```python
from build123d import *
from build123d import SkipClean  # not in build123d's __all__

# Parameters (mm, degrees)
F0_W     = 48
F0_H     = 30
F0_R     = 1.5
F0_W_2   = 14
F0_H_2   = 5
F0_W_3   = 5
F0_H_3   = 11
F0_R_2   = 3
F0_R_3   = 1.75
F1_DEPTH = 6
F2_DEPTH = 2
F5_DEPTH = 12
F6_DEPTH = 12.001
F7_DEPTH = 30.001


with BuildPart() as f1:
    # F0 (on Front) → F1 (new body)
    with BuildSketch(Plane.XZ):
        Rectangle(F0_W, F0_H)
        with Locations((-15.5, -11)):
            Circle(F0_R, mode=Mode.SUBTRACT)
        with Locations((-6, -5)):
            Rectangle(F0_W_2, F0_H_2, mode=Mode.SUBTRACT)
        with Locations((3.5, -11)):
            Circle(F0_R, mode=Mode.SUBTRACT)
        with Locations((9.5, -5.5)):
            Rectangle(F0_W_3, F0_H_3, mode=Mode.SUBTRACT)
        with Locations((-18, 8)):
            Circle(F0_R_2, mode=Mode.SUBTRACT)
        with Locations((8, 8)):
            Circle(F0_R_2, mode=Mode.SUBTRACT)
        with Locations((-6, -5)):
            Rectangle(F0_W_2, F0_H_2)
        with Locations((9.5, -5.5)):
            Rectangle(F0_W_3, F0_H_3)
        with Locations((8, 8)):
            Circle(F0_R_2)
        with Locations((8, 8)):
            Circle(F0_R_3, mode=Mode.SUBTRACT)
        with Locations((-18, 8)):
            Circle(F0_R_2)
        with Locations((-18, 8)):
            Circle(F0_R_3, mode=Mode.SUBTRACT)
    extrude(amount=-F1_DEPTH)

    # F0 (on Front) → F2 (cut)
    with BuildSketch(Plane.XZ):
        with Locations((9.5, -5.5)):
            Rectangle(F0_W_3, F0_H_3)
        with Locations((-6, -5)):
            Rectangle(F0_W_2, F0_H_2)
        with Locations((-18, 8)):
            Circle(F0_R_2)
        with Locations((-18, 8)):
            Circle(F0_R_3, mode=Mode.SUBTRACT)
        with Locations((8, 8)):
            Circle(F0_R_2)
        with Locations((8, 8)):
            Circle(F0_R_3, mode=Mode.SUBTRACT)
    extrude(amount=-F2_DEPTH, mode=Mode.SUBTRACT)

    # F4 (on face) → F5 (join)
    with BuildSketch(Plane.XY.offset(15)):
        with BuildLine():
            Line((-24, 12), (-24, 6))
            Line((-24, 6), (-11.2915026221, 6))
            ThreePointArc((-11.2915026221, 6), (-13.2915026221, 8.7084973779), (-14, 12))
            Line((-14, 12), (-24, 12))
        make_face()
        with BuildLine():
            ThreePointArc((2, 12), (1.2915026221, 8.7084973779), (-0.7084973779, 6))
            Line((-0.7084973779, 6), (24, 6))
            Line((24, 6), (24, 12))
            Line((24, 12), (2, 12))
        make_face()
    extrude(amount=-F5_DEPTH)

    # F0 (on Front) → F6 (cut, through all)
    with BuildSketch(Plane.XZ):
        with Locations((-18, 8)):
            Circle(F0_R_3)
        with Locations((8, 8)):
            Circle(F0_R_3)
    extrude(amount=-F6_DEPTH, mode=Mode.SUBTRACT)

    # F4 (on face) → F7 (cut, through all)
    with BuildSketch(Plane.XY.offset(15)):
        with BuildLine():
            Line((-0.7084973779, 6), (-11.2915026221, 6))
            ThreePointArc((-11.2915026221, 6), (-6, 4), (-0.7084973779, 6))
        make_face()
    with SkipClean():  # cleaning this boolean's faces spoils the solid; the shape is the same uncleaned
        extrude(amount=-F7_DEPTH, mode=Mode.SUBTRACT)


solid = f1.part
```
Read the model definition and answer for the solid it produces. Units are mm, in the model's axes. A direction names the side the tool comes from. Round coordinates to 2 decimals unless told otherwise and drop trailing zeros. Write each loop counter-clockwise with the first axis right and the second up, starting at its lowest first coordinate (ties: lowest second). Pieces come first, ordered by that corner, then holes. Notation, with made-up numbers: (2.5, 8.5) -> (10.5, 8.5) arc R30 cw to (10.5, 33.5) -> close; hole circle Ø10 at (9, -8.5). An arc over 180 degrees is marked (long way). Answer in a Markdown table with one row per item. Add a question column.
1) Given P1, Ø5, axis at x = -18, z = 8, coming from the -Y side; P2, Ø4, axis at x = -18, z = -7, coming from the +Y side; P3, Ø5, axis at x = -19, y = 10.5, coming from the -Z side, each flat-ended and moving along its own axis, determine where each tip first touches the part or whether it passes through.
2) Find section D-D, the plane y = 10. Determine the outline of the cut face in (x, z), and give its area (3 significant figures).
3) Determine the mould class of faces 4 (the face through (-20, 12, 9)), 5 (the face through (0, 3, -15)), 6 (the face through (-21, 1, 8)) for opening direction Z: pulls with the +Z half, pulls with the -Z half, needs draft (parallel to the pull), parting line crosses it, or undercut.
4) Consider line 1 (X direction, y = 1.5, z = -3); line 2 (Z direction, x = 8, y = 8); line 3 (Y direction, x = -17.5, z = 5.25). Determine where each line is inside the solid, lowest interval first.
5) Which of the six approach directions +Z, -Z, +X, -X, +Y, -Y give full straight-line access (tool end or side, diameter ignored) to faces 1 (the face through (11, 6, -6)), 2 (the face through (24, 5, 3)), 3 (the face through (-6, 2, -5))?
6) Find section B-B, the plane y = 4.75. Determine the outline of the cut face in (x, z), and give its area (3 significant figures).
7) Find section A-A, the plane x = -18. Determine the outline of the cut face in (y, z), and give its area (3 significant figures).
8) Find section C-C, the plane z = 9. Determine the outline of the cut face in (x, y).
Findings below:
| question | item | result |
|---|---|---|
| 1 | P1 | y = 2 |
| 1 | P2 | y = 6 |
| 1 | P3 | z = 3 |
| 2 | outline | (-24, 3) -> (-13.75, 3) -> (-13.75, 15) -> (-24, 15) -> close; (1.75, 3) -> (24, 3) -> (24, 15) -> (1.75, 15) -> close; hole circle Ø3.5 at (-18, 8); hole circle Ø3.5 at (8, 8) |
| 2 | area | 371 mm² |
| 3 | face 4 | needs draft |
| 3 | face 5 | pulls with the -Z half |
| 3 | face 6 | undercut |
| 4 | line 1 | -24 to -13, 1 to 7, 12 to 24 |
| 4 | line 2 | 3 to 6.25, 9.75 to 15 |
| 4 | line 3 | 2 to 12 |
| 5 | face 1 | -Z, +X, -X, +Y |
| 5 | face 2 | +Z, -Z, +X, +Y, -Y |
| 5 | face 3 | -Y |
| 6 | outline | (-24, -15) -> (-9.38, -15) -> (-9.38, 15) -> (-24, 15) -> close; (-2.62, -15) -> (24, -15) -> (24, 15) -> (-2.62, 15) -> close; hole circle Ø3.5 at (-18, 8); hole circle Ø3 at (-15.5, -11); hole circle Ø3 at (3.5, -11); hole circle Ø3.5 at (8, 8) |
| 6 | area | 1,200 mm² |
| 7 | outline | (0, -15) -> (6, -15) -> (6, 3) -> (12, 3) -> (12, 6.25) -> (2, 6.25) -> (2, 5) -> (0, 5) -> close; (0, 11) -> (2, 11) -> (2, 9.75) -> (12, 9.75) -> (12, 15) -> (0, 15) -> close |
| 7 | area | 205 mm² |
| 8 | outline | (-24, 0) -> (-20.83, 0) -> (-20.83, 2) -> (-19.44, 2) -> (-19.44, 12) -> (-24, 12) -> close; (-16.56, 2) -> (-15.17, 2) -> (-15.17, 0) -> (5.17, 0) -> (5.17, 2) -> (6.56, 2) -> (6.56, 12) -> (2, 12) arc R8 cw to (-14, 12) -> (-16.56, 12) -> close; (9.44, 2) -> (10.83, 2) -> (10.83, 0) -> (24, 0) -> (24, 12) -> (9.44, 12) -> close |
